Input: dimensioned drawing with shaded views. Units: mm. Origin: part minimum x, y, z. Give positions to 0.01 mm unless a question says otherwise; leave off trailing zeros. Write each loop counter-clockwise with the first axis right and the second up, starting at its lowest first coordinate (ties: lowest second). Pieces come first, ordered by that corner, then holes. Notation, with made-up numbers: (-32.5, -20) -> (2.5, -20) arc R10 cw to (2.5, -12) -> close; hole circle Ø3 at (26, 83). An arc over 180 degrees is marked (long way). Answer in a Markdown table with one row per item. Add a question column.
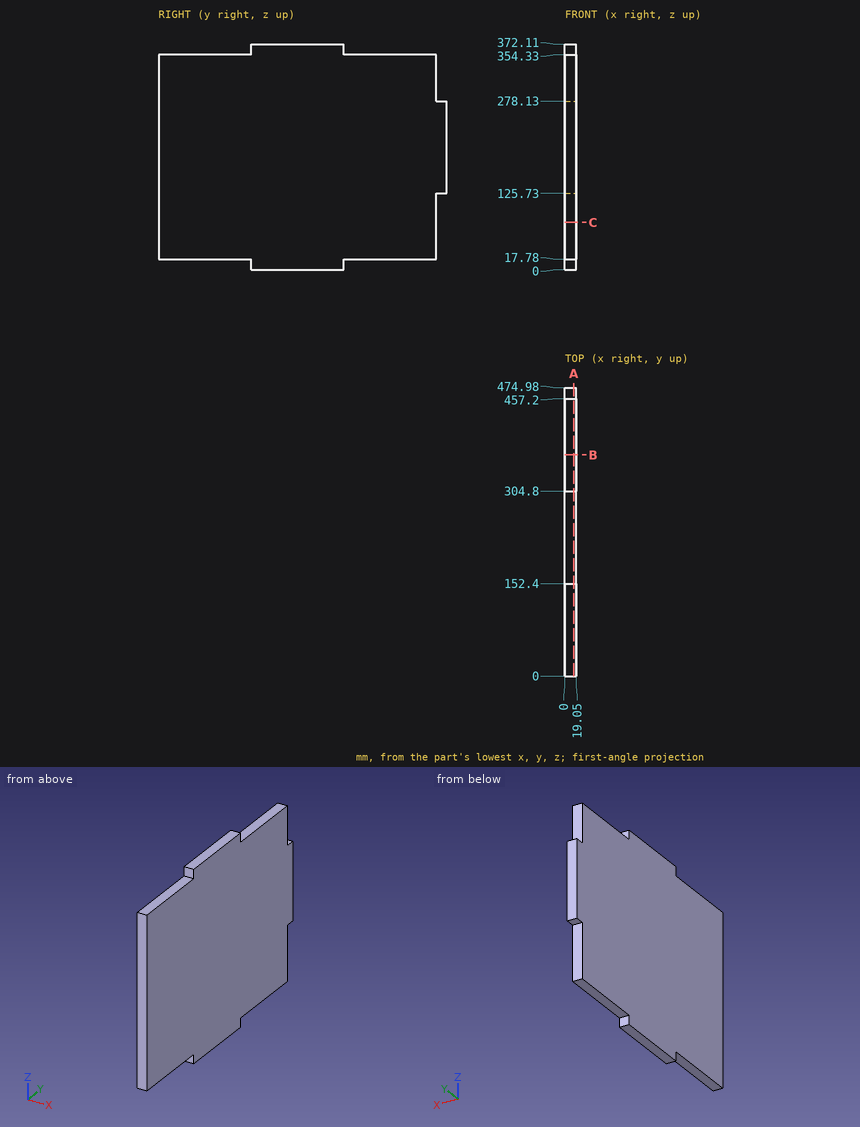
Q1. Section C-C on z = 78. Return loops of the section in (x, y), and give its area (3 significant figures).
Q2. Line query: probe 1 along Y at (x, z) = (14.75, 52); probe 2 along Z at (x, y) = (14.5, 92). Output: solid intervals per line, ascending. Write a range as from..to.
Q3. Contact query for flat-ended pins moving along their axis: pin 1 Ø8 at (x, y) = (4.5, 313) entering from -Z; pin 2 Ø9.5 at (x, z) = (7, 45) entering from +Y; pin 3 Ø6 at (x, y) = (15.5, 231.5) entering from -Z; pin 4 Ø1.5 at (x, y) = (7.5, 419) entering from +Z. Output: stop coordinate, or through.
Q4. Section A-A on x = 15. Return loops of the section in (y, z).
Q5. Section B-B on y = 364.5. Return loops of the section in (x, z).
Checks:
| question | item | result |
|---|---|---|
| 1 | outline | (0, 0) -> (19.05, 0) -> (19.05, 457.2) -> (0, 457.2) -> close |
| 1 | area | 8,710 mm^2 |
| 2 | probe 1 | 0..457.2 |
| 2 | probe 2 | 17.78..354.33 |
| 3 | pin 1 | z = 17.78 |
| 3 | pin 2 | y = 457.2 |
| 3 | pin 3 | z = 0 |
| 3 | pin 4 | z = 354.33 |
| 4 | outline | (0, 17.78) -> (152.4, 17.78) -> (152.4, 0) -> (304.8, 0) -> (304.8, 17.78) -> (457.2, 17.78) -> (457.2, 125.73) -> (474.98, 125.73) -> (474.98, 278.13) -> (457.2, 278.13) -> (457.2, 354.33) -> (304.8, 354.33) -> (304.8, 372.11) -> (152.4, 372.11) -> (152.4, 354.33) -> (0, 354.33) -> close |
| 5 | outline | (0, 17.78) -> (19.05, 17.78) -> (19.05, 354.33) -> (0, 354.33) -> close |
